Work out the finished part from the listing and answer in its coordinate system (mm). Face numbers are marked on the shaded views. A direction names the side the tool comes from. Round coordinates to 2 decimals unless told otherwise and drop trailing zeros. Order: outer loops, then holes, each group sorted by start corner. A loop starts at its lowest first (then second) coordinate and runs counter-clockwise, first axis right, second up. Notation, with made-up numbers: M 57.25,70 L 104.25,70 A26 cw 104.25,88 Z; hole C 53.25,63.25 d2. An arc over 180 degrees is marked long. Return JSON: item names as keys, results as strings.
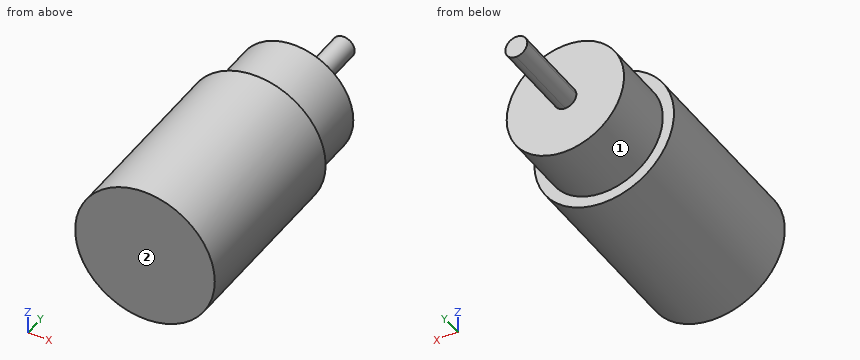
from build123d import *

# Parameters (mm, degrees)
F0_R     = 16
F1_DEPTH = 17.78
F2_R     = 19.05
F3_DEPTH = 50.8
F5_DEPTH = 22.479


with BuildPart() as f1:
    # F0 (on Front) → F1 (new body)
    with BuildSketch(Plane.XZ):
        Circle(F0_R)
    extrude(amount=F1_DEPTH)

    # F2 (on face) → F3 (join)
    with BuildSketch(Plane.XZ.offset(17.78)):
        Circle(F2_R)
    extrude(amount=F3_DEPTH)

    # F4 (on face) → F5 (join)
    with BuildSketch(Plane(origin=(0, 0, 0), x_dir=(-1, 0, 0), z_dir=(0, 1, 0))):
        with BuildLine():
            ThreePointArc((0, -3), (2.12132, -2.12132), (3, 0))
            ThreePointArc((3, 0), (-2.12132, 2.12132), (0, -3))
        make_face()
    extrude(amount=F5_DEPTH)


solid = f1.part
Item 1: Find section A-A (x = 5). Determine the outline of the cut face in (y, z).
Output:
{"outline": "M -68.58,-18.38 L -17.78,-18.38 L -17.78,-15.2 L 0,-15.2 L 0,15.2 L -17.78,15.2 L -17.78,18.38 L -68.58,18.38 Z"}
Item 2: Find section C-C (y = -13.5). Determine the outline of the cut face in (x, z).
Output:
{"outline": "C 0,0 d32"}
Item 3: Consider line 1 along Y through (x, z) = (-0.5, 7.5); line 2 along Z through (x, y) = (-0.5, -12.5); line 3 along Y through (x, z) = (-10.5, -14). Determine where each line is inside the solid, lowest interval first. Write a range as [from, to].
Output:
{"line 1": "y = [-68.58, 0]", "line 2": "z = [-15.99, 15.99]", "line 3": "y = [-68.58, -17.78]"}
Item 4: Find section D-D (y = -46). Determine the outline of the cut face in (x, z).
Output:
{"outline": "C 0,0 d38.1"}
Item 5: Each of these flat-tipped pins is pushed along its axis until it touches: pin 1 (5 mm diameter, centred on x = 14.5, z = 14, fed in from +Y); pin 2 (5 mm diameter, centred on x = 11, y = -33, fed in from +Z); pin 3 (12 mm diameter, centred on x = 13, z = 6, fed in from +Y). Where does it stop, or does it pass through?
Output:
{"pin 1": "stops at y = -17.78", "pin 2": "stops at z = 17.05", "pin 3": "stops at y = 0"}
Item 6: Find section B-B (z = -13). Determine the outline of the cut face in (x, y).
Output:
{"outline": "M -13.92,-68.58 L 13.92,-68.58 L 13.92,-17.78 L 9.33,-17.78 L 9.33,0 L -9.33,0 L -9.33,-17.78 L -13.92,-17.78 Z"}
Item 7: Which of the six approach directions +Z, -Z, +X, -X, +Y, -Y give full straight-line access (tool end or side, diameter ignored) to the marked faces 1 and 2?
Output:
{"face 1": "+Y", "face 2": "+Z, -Z, +X, -X, -Y"}
